from build123d import *


with BuildPart() as f1:
    # F0 (on Front) → F1 (revolve)
    with BuildSketch(Plane.XZ):
        with BuildLine():
            Line((0, 2.570061), (0, 0))
            Line((0, 0), (38.1, 0))
            Line((38.1, 0), (38.1, 2.250872))
            ThreePointArc((38.1, 2.250872), (36.834626, 7.301015), (33.3375, 11.157857))
            Line((33.3375, 11.157857), (33.3375, 4.784073))
            Line((33.3375, 4.784073), (6.203805, 4.784073))
            Line((6.203805, 4.784073), (6.203805, 8.688359))
            ThreePointArc((6.203805, 8.688359), (1.822309, 6.926687), (0, 2.570061))
        make_face()
    revolve(axis=Axis((19.05, 0, 0), (1, 0, 0)))


solid = f1.part
The model under review builds one solid part; all positions refer to its coordinate system, in mm. Round coordinates to 2 decimals unless told otherwise and drop trailing zeros. Order: outer loops, then holes, each group sorted by start corner. A loop starts at its lowest first (then second) coordinate and runs counter-clockwise, first axis right, second up. Notation, with made-up numbers: (67, 39) -> (79, 39) arc R27 ccw to (79, 62) -> close; hole circle Ø9 at (-24, 42). An arc over 180 degrees is marked (long way). Return JSON: item names as keys, results as strings.
1. The part is to be moulded in two halves that separate along X. For faces 1 (the face through (19.581, 4.244, 2.208)), 2 (the face through (38.1, 0, 0)), 3 (the face through (0, 0, 0)), say which applies: +X half, -X half, draft (parallel to the pull), parting line (faces both ways), or undercut.
Answer block:
{"face 1": "undercut", "face 2": "+X half", "face 3": "-X half"}
2. For L1, parallel to X at y = 1.75, z = -6.25; L2, parallel to X at y = 5.25, z = 3; L3, parallel to Z at x = 16, y = 4, list the stretches that pass through material, from the lowest coordinate up. Write a range as [from, to].
Answer block:
{"L1": "x = [1.42, 6.2], [33.34, 37.23]", "L2": "x = [1.08, 6.2], [33.34, 37.4]", "L3": "z = [-2.62, 2.62]"}
3. Insertion check: P1, Ø1.5, axis at x = 14.5, z = -7, coming from the -Y side; P2, Ø2, axis at y = 5, z = -1.5, coming from the -X side; P3, Ø8, axis at x = 14.5, y = -3, coming from the +Z side; P4, Ø5, axis at y = 6.5, z = -5.5, coming from the +X side. Each pin has a flat end and moves straight along its axis. Give the tip position at first contact, or say it passes through.
Answer block:
{"P1": "passes through", "P2": "stops at x = 0.23", "P3": "stops at z = 4.78", "P4": "stops at x = 37.42"}
4. Take a section at A-A (x = 13). Write out the cut boundary in (y, z), then the cut area to 3 significant figures.
Answer block:
{"outline": "circle Ø9.57 at (0, 0)", "area": "71.9 mm²"}
